```python
from build123d import *

# Parameters (mm, degrees)
SKETCH1_R           = 2.5
SKETCH1_R_2         = 1.1
BOSS_EXTRUDE1_DEPTH = 7
BOSS_EXTRUDE2_REACH = 52
SKETCH2_W           = 0.9
SKETCH2_H           = 6.1
CUT_EXTRUDE1_REACH  = 2.9
SKETCH3_R           = 2.5


with BuildPart() as part:
    # Sketch1 → Boss-Extrude1 (new body)
    with BuildSketch(Plane.XY):
        with BuildLine():
            Line((3, 0), (17, 0))
            ThreePointArc((17, 0), (19.121320344, 0.878679656), (20, 3))
            Line((20, 3), (20, 14.92820323))
            Line((20, 14.92820323), (28.124355653, 29))
            Line((28.124355653, 29), (47, 29))
            ThreePointArc((47, 29), (49.121320344, 29.878679656), (50, 32))
            Line((50, 32), (50, 45))
            ThreePointArc((50, 45), (49.121320344, 47.121320344), (47, 48))
            Line((47, 48), (17.732050808, 48))
            ThreePointArc((17.732050808, 48), (16.232050808, 47.598076211), (15.133974596, 46.5))
            Line((15.133974596, 46.5), (0.401923789, 20.983339502))
            ThreePointArc((0.401923789, 20.983339502), (0.102222521, 20.259796637), (0, 19.483339502))
            Line((0, 19.483339502), (0, 3))
            ThreePointArc((0, 3), (0.878679656, 0.878679656), (3, 0))
        make_face()
        with Locations((20, 39)):
            Circle(SKETCH1_R, mode=Mode.SUBTRACT)
        with Locations((40, 39)):
            Circle(SKETCH1_R, mode=Mode.SUBTRACT)
        with Locations((10, 5.4)):
            Circle(SKETCH1_R_2, mode=Mode.SUBTRACT)
        with Locations((10, 15)):
            Circle(SKETCH1_R_2, mode=Mode.SUBTRACT)
    extrude(amount=BOSS_EXTRUDE1_DEPTH)

    # Boss-Extrude2: up to this face of the body (flat: up to its plane)
    boss_extrude2_end = Plane(part.part.faces().sort_by_distance((7.767949192, 33.741669751, 3.5))[0])
    # Sketch2 → Boss-Extrude2 (add, up to the picked face)
    with BuildSketch(Plane(origin=(50, 0, 0), x_dir=(0, 0, -1), z_dir=(1, 0, 0)), mode=Mode.PRIVATE) as boss_extrude2_sk1:
        with Locations((0.45, 39)):
            Rectangle(SKETCH2_W, SKETCH2_H)
    boss_extrude2_tool1 = split(extrude(boss_extrude2_sk1.sketch, amount=-BOSS_EXTRUDE2_REACH, mode=Mode.PRIVATE), bisect_by=boss_extrude2_end, keep=Keep.BOTH, mode=Mode.PRIVATE)
    add(boss_extrude2_tool1.solids().sort_by_distance((50, 39, -0.45))[0])

    # Sketch3 → Cut-Extrude1 (cut, up to next)
    with BuildSketch(Plane.XY, mode=Mode.PRIVATE) as cut_extrude1_sk1:
        with Locations((20, 39)):
            Circle(SKETCH3_R)
    cut_extrude1_tool1 = extrude(cut_extrude1_sk1.sketch, amount=-CUT_EXTRUDE1_REACH, mode=Mode.PRIVATE) & part.part
    add(cut_extrude1_tool1.solids().sort_by_distance((20, 39, 0))[0], mode=Mode.SUBTRACT)
    # Sketch3 → Cut-Extrude1 (cut, up to next)
    with BuildSketch(Plane.XY, mode=Mode.PRIVATE) as cut_extrude1_sk2:
        with Locations((40, 39)):
            Circle(SKETCH3_R)
    cut_extrude1_tool2 = extrude(cut_extrude1_sk2.sketch, amount=-CUT_EXTRUDE1_REACH, mode=Mode.PRIVATE) & part.part
    add(cut_extrude1_tool2.solids().sort_by_distance((40, 39, 0))[0], mode=Mode.SUBTRACT)


solid = part.part
```
For this review, take the finished solid that the model builds, in its own axes (mm). A direction names the side the tool comes from. Round coordinates to 2 decimals unless told otherwise and drop trailing zeros. Loops run counter-clockwise (first coordinate to the right, second up) from the corner with the lowest first, then second, coordinate; pieces in that order, holes last.
Q1. To check wall thickness, follow line 1 along Y through (x, z) = (40, -0.7); line 2 along Y through (x, z) = (40, 3); line 3 along Y through (x, z) = (10, 3.5). State the ranges of each line that lie inside material, in increasing order.
Result sheet:
line 1: y = 35.95 to 36.5, 41.5 to 42.05
line 2: y = 29 to 36.5, 41.5 to 48
line 3: y = 0 to 4.3, 6.5 to 13.9, 16.1 to 37.61
Q2. Add section D-D on y = 39. Write out the cut boundary in (x, z).
Result sheet:
outline: (10.8, -0.9) - (17.5, -0.9) - (17.5, 7) - (10.8, 7) - close; (22.5, -0.9) - (37.5, -0.9) - (37.5, 7) - (22.5, 7) - close; (42.5, -0.9) - (50, -0.9) - (50, 7) - (42.5, 7) - close
Q3. Add section B-B on x = 40. Write out the cut boundary in (y, z), plus the area to 3 significant figures.
Result sheet:
outline: (29, 0) - (35.95, 0) - (35.95, -0.9) - (36.5, -0.9) - (36.5, 7) - (29, 7) - close; (41.5, -0.9) - (42.05, -0.9) - (42.05, 0) - (48, 0) - (48, 7) - (41.5, 7) - close
area: 99.0 mm2
Q4. Add section C-C on x = 32.5. Write out the cut boundary in (y, z), plus the area to 3 significant figures.
Result sheet:
outline: (29, 0) - (35.95, 0) - (35.95, -0.9) - (42.05, -0.9) - (42.05, 0) - (48, 0) - (48, 7) - (29, 7) - close
area: 138 mm2
Q5. Add section A-A on z = 1. Write out the cut boundary in (x, y).
Result sheet:
outline: (0, 3) arc R3 ccw to (3, 0) - (17, 0) arc R3 ccw to (20, 3) - (20, 14.93) - (28.12, 29) - (47, 29) arc R3 ccw to (50, 32) - (50, 45) arc R3 ccw to (47, 48) - (17.73, 48) arc R3 ccw to (15.13, 46.5) - (0.4, 20.98) arc R3 ccw to (0, 19.48) - close; hole circle Ø2.2 at (10, 5.4); hole circle Ø2.2 at (10, 15); hole circle Ø5 at (20, 39); hole circle Ø5 at (40, 39)
Q6. Machinability: for faces 1 (the face through (37, 29, 3)), 2 (the face through (19, 22, 0)), 3 (the face through (31, 45, 0)), which of the approach directions +Z, -Z, +X, -X, +Y, -Y give a long, thin tool a straight path to every point of the face, cutting with its end or side? Answer none if there is none.
Result sheet:
face 1: +Z, -Z, +X, -Y
face 2: -Z, +X, -X, -Y
face 3: -Z, +X, -X, +Y
Q7. Insertion check: pin 1 Ø3 at (x, y) = (27, 45) entering from -Z; pin 2 Ø1.5 at (y, z) = (14, 0) entering from +X; pin 3 Ø3.5 at (x, z) = (38, 3.5) entering from -Y. Each pin has a flat end and moves straight along its axis. Give the tip position at first contact, or say it passes through.
Result sheet:
pin 1: stops at z = 0
pin 2: stops at x = 20
pin 3: stops at y = 29
